```python
from build123d import *

# Parameters (mm, degrees)
SKETCH_1_W      = 23
SKETCH_1_H      = 13
SKETCH_1_R      = 1
SKETCH_1_R_2    = 1.5
EXTRUDE_1_DEPTH = 2
FILLET_1_R      = 1


with BuildPart() as part:
    # 草图1 → 凸台-拉伸1 (new body)
    with BuildSketch(Plane.XY):
        Rectangle(SKETCH_1_W, SKETCH_1_H)
        with Locations((-9.5, 4)):
            Circle(SKETCH_1_R, mode=Mode.SUBTRACT)
        with Locations((-9.5, -4)):
            Circle(SKETCH_1_R, mode=Mode.SUBTRACT)
        with Locations(Location((9.5, -4, 0), (0, 0, 180))):
            Circle(SKETCH_1_R, mode=Mode.SUBTRACT)
        with Locations(Location((9.5, 4, 0), (0, 0, 180))):
            Circle(SKETCH_1_R, mode=Mode.SUBTRACT)
        Circle(SKETCH_1_R_2, mode=Mode.SUBTRACT)
    extrude(amount=EXTRUDE_1_DEPTH)

    # 圆角1
    fillet_1_edges = [part.edges().sort_by_distance(p)[0] for p in [
        (11.5, -6.5, 1),
        (-11.5, -6.5, 1),
        (-11.5, 6.5, 1),
        (11.5, 6.5, 1),
    ]]
    fillet(fillet_1_edges, radius=FILLET_1_R)


solid = part.part
```
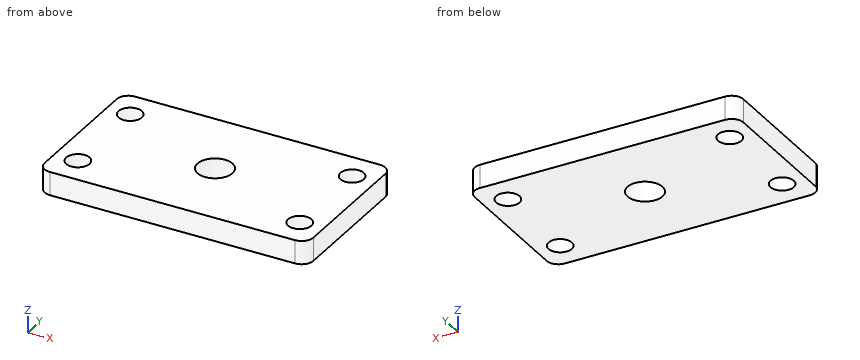
Verification items for the finished model (mm, model axes). Coordinates: 2 decimals unless noted, no trailing zeros. Write each loop counter-clockwise with the first axis right and the second up, starting at its lowest first coordinate (ties: lowest second). Pieces come first, ordered by that corner, then holes. Notation, with made-up numbers: M -8.5,70 L 7.5,70 A22 cw 7.5,83 Z; hole C -4.5,88 d10. An arc over 180 degrees is marked long. One line per item, written item: value.
Item 1: Section check A-A, the plane y = 0. Record the boundary of the cut face in (x, z), plus the area to 3 significant figures.
Check sheet entries:
outline: M -11.5,0 L -1.5,0 L -1.5,2 L -11.5,2 Z; M 1.5,0 L 11.5,0 L 11.5,2 L 1.5,2 Z
area: 40.0 mm^2
Item 2: Section check B-B, the plane x = -9.5. Record the boundary of the cut face in (y, z), plus the area to 3 significant figures.
Check sheet entries:
outline: M -6.5,0 L -5,0 L -5,2 L -6.5,2 Z; M -3,0 L 3,0 L 3,2 L -3,2 Z; M 5,0 L 6.5,0 L 6.5,2 L 5,2 Z
area: 18.0 mm^2
Item 3: Scan lines: line 1 along Y through (x, z) = (9.5, 1.25); line 2 along X through (y, z) = (3.5, 0.55); line 3 along X through (y, z) = (-4.75, 1.95). Record each from-to range of solid material in increasing order.
Check sheet entries:
line 1: y = -6.5 to -5, -3 to 3, 5 to 6.5
line 2: x = -11.5 to -10.37, -8.63 to 8.63, 10.37 to 11.5
line 3: x = -11.5 to -10.16, -8.84 to 8.84, 10.16 to 11.5
Item 4: Section check C-C, the plane z = 1.25. Record the boundary of the cut face in (x, y), plus the area to 3 significant figures.
Check sheet entries:
outline: M -11.5,-5.5 A1 ccw -10.5,-6.5 L 10.5,-6.5 A1 ccw 11.5,-5.5 L 11.5,5.5 A1 ccw 10.5,6.5 L -10.5,6.5 A1 ccw -11.5,5.5 Z; hole C -9.5,-4 d2; hole C -9.5,4 d2; hole C 0,0 d3; hole C 9.5,-4 d2; hole C 9.5,4 d2
area: 279 mm^2
Item 5: Gauge pin test, flat end, axial feed: pin 1 Ø1.2 at (x, y) = (9.5, 4) entering from +Z. Record the tip position at first contact, or that the pin passes through.
Check sheet entries:
pin 1: passes through
Item 6: Section check D-D, the plane y = -4. Record the boundary of the cut face in (x, z).
Check sheet entries:
outline: M -11.5,0 L -10.5,0 L -10.5,2 L -11.5,2 Z; M -8.5,0 L 8.5,0 L 8.5,2 L -8.5,2 Z; M 10.5,0 L 11.5,0 L 11.5,2 L 10.5,2 Z
